```python
from build123d import *

# Parameters (mm, degrees)
BOSS_EXTRUDE1_DEPTH                            = 3
CSK_FOR_M3_FLAT_HEAD_MACHINE_SCREW1_AT_2_COUNT = 2
CSK_FOR_M3_FLAT_HEAD_MACHINE_SCREW1_AT_2_PITCH = 204
CSK_FOR_M3_FLAT_HEAD_MACHINE_SCREW1_AT_3_COUNT = 2
CSK_FOR_M3_FLAT_HEAD_MACHINE_SCREW1_AT_3_PITCH = 288.499566724
CSK_FOR_M3_FLAT_HEAD_MACHINE_SCREW1_AT_4_COUNT = 2
CSK_FOR_M3_FLAT_HEAD_MACHINE_SCREW1_AT_4_PITCH = 204
BOSS_EXTRUDE2_START                            = -3
BOSS_EXTRUDE2_DEPTH                            = 8
SKETCH6_W                                      = 24
SKETCH6_H                                      = 7
CUT_EXTRUDE1_DEPTH                             = 6


with BuildPart() as part:
    # Sketch1 → Boss-Extrude1 (new body)
    with BuildSketch(Plane(origin=(0, 0, 0), x_dir=(1, 0, 0), z_dir=(0, 1, 0))):
        with BuildLine():
            Line((-106, 109), (106, 109))
            ThreePointArc((106, 109), (108.121320344, 108.121320344), (109, 106))
            Line((109, 106), (109, -106))
            ThreePointArc((109, -106), (108.121320344, -108.121320344), (106, -109))
            Line((106, -109), (-106, -109))
            ThreePointArc((-106, -109), (-108.121320344, -108.121320344), (-109, -106))
            Line((-109, -106), (-109, 106))
            ThreePointArc((-109, 106), (-108.121320344, 108.121320344), (-106, 109))
        make_face()
    extrude(amount=BOSS_EXTRUDE1_DEPTH)

    # Sketch4 → CSK for M3 Flat Head Machine Screw1 (revolve, cut)
    with BuildSketch(Plane(origin=(-102, 3, -102), x_dir=(0, 0, 1), z_dir=(1, 0, 0))):
        Polygon((0, 0), (0, 3), (1.7, 3), (1.7, 1.45), (3.15, 0), align=None)
    csk_for_m3_flat_head_machine_screw1 = revolve(axis=Axis((-102, 9.35, -102), (0, -1, 0)), mode=Mode.SUBTRACT)

    # CSK for M3 Flat Head Machine Screw1 at 2: CSK for M3 Flat Head Machine Screw1 ×2
    with Locations(*[(0, 0, i * CSK_FOR_M3_FLAT_HEAD_MACHINE_SCREW1_AT_2_PITCH) for i in range(1, CSK_FOR_M3_FLAT_HEAD_MACHINE_SCREW1_AT_2_COUNT)]):
        add(csk_for_m3_flat_head_machine_screw1, mode=Mode.SUBTRACT)

    # CSK for M3 Flat Head Machine Screw1 at 3: CSK for M3 Flat Head Machine Screw1 ×2
    with Locations(*[Vector(0.7071067811865476, 0, 0.7071067811865475) * (i * CSK_FOR_M3_FLAT_HEAD_MACHINE_SCREW1_AT_3_PITCH) for i in range(1, CSK_FOR_M3_FLAT_HEAD_MACHINE_SCREW1_AT_3_COUNT)]):
        add(csk_for_m3_flat_head_machine_screw1, mode=Mode.SUBTRACT)

    # CSK for M3 Flat Head Machine Screw1 at 4: CSK for M3 Flat Head Machine Screw1 ×2
    with Locations(*[(i * CSK_FOR_M3_FLAT_HEAD_MACHINE_SCREW1_AT_4_PITCH, 0, 0) for i in range(1, CSK_FOR_M3_FLAT_HEAD_MACHINE_SCREW1_AT_4_COUNT)]):
        add(csk_for_m3_flat_head_machine_screw1, mode=Mode.SUBTRACT)

    # Sketch5 → Boss-Extrude2 (add)
    with BuildSketch(Plane(origin=(0, 0, 0), x_dir=(-1, 0, 0), z_dir=(0, -1, 0)).offset(BOSS_EXTRUDE2_START)):
        Polygon((0, 109), (12, 109), (12, 119), (-12, 119), (-12, 109), align=None)
    extrude(amount=BOSS_EXTRUDE2_DEPTH)

    # Sketch6 → Cut-Extrude1 (cut)
    with BuildSketch(Plane(origin=(0, 3, 0), x_dir=(1, 0, 0), z_dir=(0, 1, 0))):
        with Locations((0, 115.5)):
            Rectangle(SKETCH6_W, SKETCH6_H)
    extrude(amount=-CUT_EXTRUDE1_DEPTH, mode=Mode.SUBTRACT)


solid = part.part
```
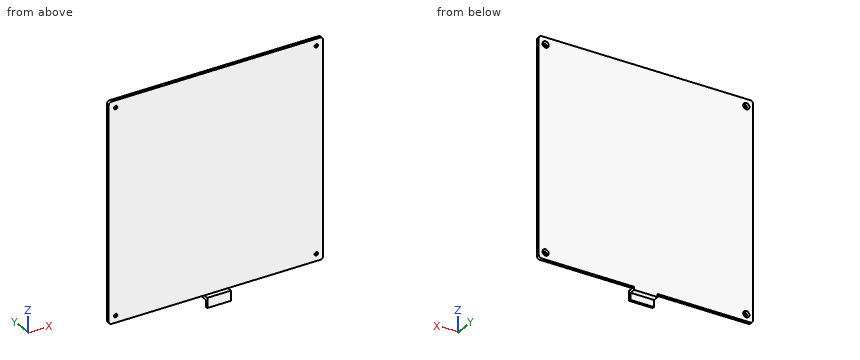
Check sheet for the modelled part. Datum: model origin and axes. Units: mm. Round coordinates to 2 decimals unless told otherwise and drop trailing zeros. Order: outer loops, then holes, each group sorted by start corner. A loop starts at its lowest first (then second) coordinate and runs counter-clockwise, first axis right, second up. Notation, with made-up numbers: (3.5, -0.5) - (10.5, -0.5) arc R11 ccw to (10.5, 12.5) - close; hole circle Ø11 at (63.25, 45.5). An arc over 180 degrees is marked (long way). Write item = value, one per line.
Q1. Section check A-A (x = -18). Record the boundary of the cut face in (y, z), and give its area (3 significant figures).
Computed:
outline = (0, -109) - (3, -109) - (3, 109) - (0, 109) - close
area = 654 mm^2
Q2. Section check B-B (z = 69.5). Record the boundary of the cut face in (x, y).
Computed:
outline = (-109, 0) - (109, 0) - (109, 3) - (-109, 3) - close
Q3. Go/stop test with flat-tipped pins: pin 1 (4 mm diameter, centred on x = -102, z = -102, fed in from -Y); pin 2 (1.5 mm diameter, centred on y = -1, z = 26, fed in from +X); pin 3 (3.5 mm diameter, centred on x = 49.5, y = 2, fed in from -Z); pin 4 (3 mm diameter, centred on x = 0.5, y = 1, fed in from -Z). Record where each tip stops, or that it passes through.
Computed:
pin_1 = 0
pin_2 = through
pin_3 = -109
pin_4 = -112
Q4. Thickness scan on line 1 along Z through (x, y) = (-102, 0.5); line 2 along Y through (x, z) = (42, -38). Record the ranges inside material, lowest first.
Computed:
line_1 = -109 to -103.7, -100.3 to 100.3, 103.7 to 109
line_2 = 0 to 3
